```python
from build123d import *

# Parameters (mm, degrees)
F0_W     = 110
F0_H     = 140
F1_DEPTH = 3.5
F3_DEPTH = 25
F5_DEPTH = 25


with BuildPart() as f1:
    # F0 (on Top) → F1 (new body)
    with BuildSketch(Plane.XY):
        Rectangle(F0_W, F0_H)
    extrude(amount=F1_DEPTH)

    # F2 (on face) → F3 (cut)
    with BuildSketch(Plane.XY.offset(3.5)):
        with BuildLine():
            ThreePointArc((-55, 20.325035), (-35.554564, 28.379598), (-27.5, 47.825035))
            ThreePointArc((-27.5, 47.825035), (-30.469277, 60.254582), (-38.735901, 70))
            Line((-38.735901, 70), (-55, 70))
            Line((-55, 70), (-55, 20.325035))
        make_face()
        with BuildLine():
            Line((-55, 70), (-38.735901, 70))
            ThreePointArc((-38.735901, 70), (-81.134857, 56.381858), (-55, 20.325035))
            Line((-55, 20.325035), (-55, 70))
        make_face()
        with BuildLine():
            ThreePointArc((-27.5, -48.937567), (-35.554564, -29.49213), (-55, -21.437567))
            Line((-55, -21.437567), (-55, -70))
            Line((-55, -70), (-37.318826, -70))
            ThreePointArc((-37.318826, -70), (-30.075291, -60.556898), (-27.5, -48.937567))
        make_face()
        with BuildLine():
            Line((-55, -70), (-55, -21.437567))
            ThreePointArc((-55, -21.437567), (-80.840539, -58.34589), (-37.318826, -70))
            Line((-37.318826, -70), (-55, -70))
        make_face()
        with BuildLine():
            ThreePointArc((82.5, 47.825035), (67.429547, 72.355757), (38.735901, 70))
            Line((38.735901, 70), (55, 70))
            Line((55, 70), (55, 20.325035))
            ThreePointArc((55, 20.325035), (74.445436, 28.379598), (82.5, 47.825035))
        make_face()
        with BuildLine():
            Line((55, 70), (38.735901, 70))
            ThreePointArc((38.735901, 70), (28.865143, 39.268211), (55, 20.325035))
            Line((55, 20.325035), (55, 70))
        make_face()
        with BuildLine():
            Line((55, -70), (55, -21.437567))
            ThreePointArc((55, -21.437567), (29.159461, -39.529244), (37.318826, -70))
            Line((37.318826, -70), (55, -70))
        make_face()
        with BuildLine():
            ThreePointArc((82.5, -48.937567), (74.445436, -29.49213), (55, -21.437567))
            Line((55, -21.437567), (55, -70))
            Line((55, -70), (37.318826, -70))
            ThreePointArc((37.318826, -70), (66.619331, -73.862276), (82.5, -48.937567))
        make_face()
    extrude(amount=-F3_DEPTH, mode=Mode.SUBTRACT)

    # F4 (on face) → F5 (cut)
    with BuildSketch(Plane.XY.offset(3.5)):
        Polygon((-60.47887, 76.34218), (-39.233364, 56.513041), (-26.769334, 76.34218), align=None)
        Polygon((26.769334, 76.34218), (39.233364, 56.513041), (60.47887, 76.34218), align=None)
        Polygon((-39.233364, -56.513041), (-60.47887, -76.34218), (-26.769334, -76.34218), align=None)
        Polygon((60.47887, -76.34218), (39.233364, -56.513041), (26.769334, -76.34218), align=None)
    extrude(amount=-F5_DEPTH, mode=Mode.SUBTRACT)


solid = f1.part
```
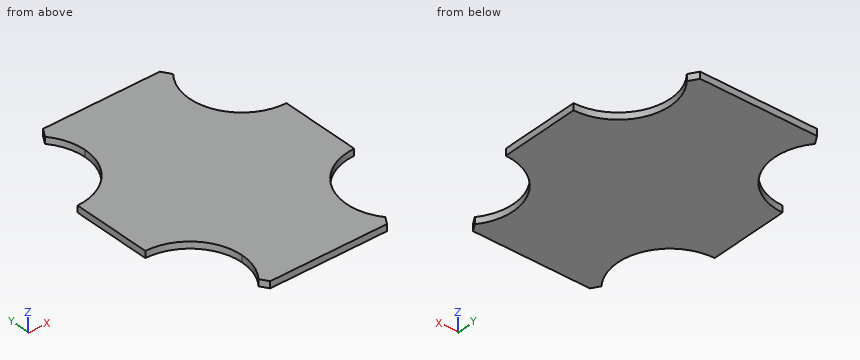
The model under review builds one solid part; all positions refer to its coordinate system, in mm. Round coordinates to 2 decimals unless told otherwise and drop trailing zeros. Loops run counter-clockwise (first coordinate to the right, second up) from the corner with the lowest first, then second, coordinate; pieces in that order, holes last. Notation, with made-up numbers: (64, 32.5) - (119, 32.5) arc R10 cw to (119, 49.5) - close; hole circle Ø11 at (4.5, -17.75). An arc over 180 degrees is marked (long way). Write each question's results on one line, items separated by ' | '. Start each with the question number.
Q1. Take a section at C-C on x = 38. Give the boundary of the cut face in (y, z).
Q2. Insertion check: P1, Ø10, axis at x = 29.5, y = 48.5, coming from the +Z side. The pin has a flat end and moves straight along its axis. Give the tip position at first contact, or say it passes through.
Q3. Wall thickness on line 1 along X through (y, z) = (63.5, 2.05); line 2 along X through (y, z) = (60, 2.5); line 3 along Y through (x, z) = (47.5, 2.55): over which ranges is each line inside the solid? List them lowest first. Write a range as [from, to].
Q4. Take a section at A-A on z = 1. Give the boundary of the cut face in (x, y).
Q5. Take a section at B-B on y = -42.5. Give the boundary of the cut face in (x, z).
Data:
1) outline: (-27.32, 0) - (26.21, 0) - (26.21, 3.5) - (-27.32, 3.5) - close
2) P1: stops at z = 3.5
3) line 1: x = [-32.4, 32.4] | line 2: x = [-30.34, 30.34] | line 3: y = [-22.48, 21.37]
4) outline: (-55, -21.44) arc R27.5 cw to (-27.5, -48.94) arc R27.5 cw to (-33.34, -65.88) - (-30.76, -70) - (30.76, -70) - (33.34, -65.88) arc R27.5 cw to (55, -21.44) - (55, 20.33) arc R27.5 cw to (33.73, 65.26) - (30.76, 70) - (-30.76, 70) - (-33.73, 65.26) arc R27.5 cw to (-27.5, 47.83) arc R27.5 cw to (-55, 20.33) - close
5) outline: (-28.26, 0) - (28.26, 0) - (28.26, 3.5) - (-28.26, 3.5) - close
